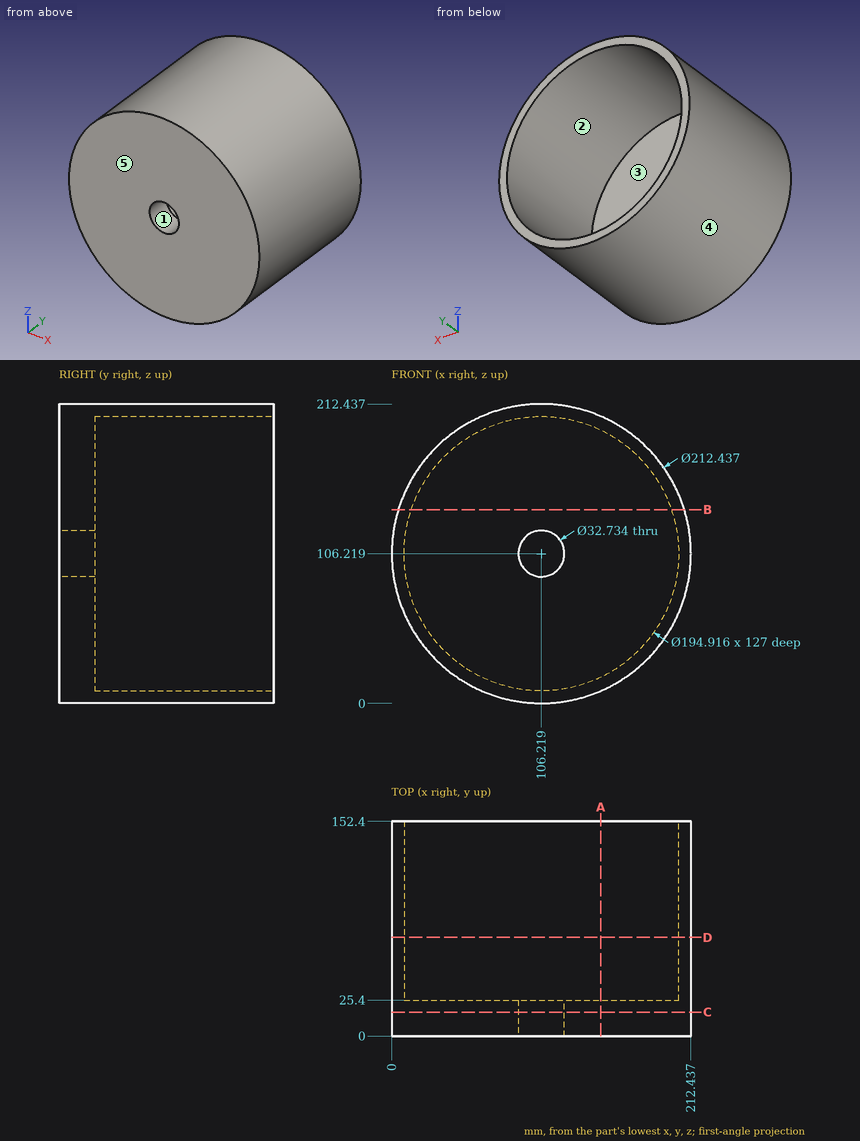
Can you work these out from the drawing? Everything is in mm from the part's minimum corner. A direction names the side the tool comes from. Give positions to 0.01 mm unless a question says otherwise; leave off trailing zeros. Order: outer loops, then holes, each group sorted by start corner. A loop starts at its lowest first (then second) coordinate and runs counter-clockwise, first axis right, second up.
Item 1: If we section it at B-B, the plane z = 137.5: Write out the boundary of the cut face in (x, y).
Item 2: If we section it at C-C, the plane y = 17: Write out the boundary of the cut face in (x, z) (1 decimal).
Item 3: If we section it at A-A, the plane x = 148.5: Write out the boundary of the cut face in (y, z), plus the area to 3 significant figures.
Item 4: If we mould it in two halves opening along Z, with no side actions, what happens to the marked faces 3, 4 and 5? For each: pulls with the +Z half, pulls with the -Z half, needs draft (parallel to the pull), parting line crosses it, or undercut.
Item 5: For the marked faces 1 and 2, which set-ups out of +Z, -Z, +X, -X, +Y, -Y let a thin tool reach every point of the face, with its end or its side?
Item 6: I need wall thicknesses on line 1 (Y direction, x = 128, z = 173); line 2 (Z direction, x = 158, y = 54) (1 decimal); line 3 (Z direction, x = 112.5, y = 114.5) (1 decimal). Which ranges of each line are inside material? Lowest first, please.
Item 7: I'm going to push flat-ended pins straight in: pin 1 (5 mm diameter, centred on x = 141, z = 114, fed in from +Y); pin 2 (10 mm diameter, centred on y = 41, z = 94.5, fed in from -X); pin 3 (6 mm diameter, centred on y = 36, z = 147, fed in from -X); pin 4 (12 mm diameter, centred on x = 140, z = 149.5, fed in from -Y). Where does each tip first touch, or does it pass through?
Item 8: If we section it at D-D, the plane y = 70: Write out the boundary of the cut face in (x, z).
Values:
1. outline: (4.71, 0) - (207.73, 0) - (207.73, 152.4) - (198.52, 152.4) - (198.52, 25.4) - (13.92, 25.4) - (13.92, 152.4) - (4.71, 152.4) - close
2. outline: circle Ø212.4 at (106.2, 106.2); hole circle Ø32.7 at (106.2, 106.2)
3. outline: (0, 8.78) - (152.4, 8.78) - (152.4, 18.41) - (25.4, 18.41) - (25.4, 194.03) - (152.4, 194.03) - (152.4, 203.66) - (0, 203.66) - close
3. area: 7,400 mm2
4. face 3: undercut
4. face 4: parting line crosses it
4. face 5: needs draft
5. face 1: +Y, -Y
5. face 2: +Y
6. line 1: y = 0 to 25.4
6. line 2: z = 13.5 to 23.7, 188.8 to 199
6. line 3: z = 0.2 to 9, 203.5 to 212.3
7. pin 1: stops at y = 25.4
7. pin 2: stops at x = 0.21
7. pin 3: stops at x = 6.95
7. pin 4: stops at y = 0
8. outline: circle Ø212.44 at (106.22, 106.22); hole circle Ø194.92 at (106.22, 106.22)
